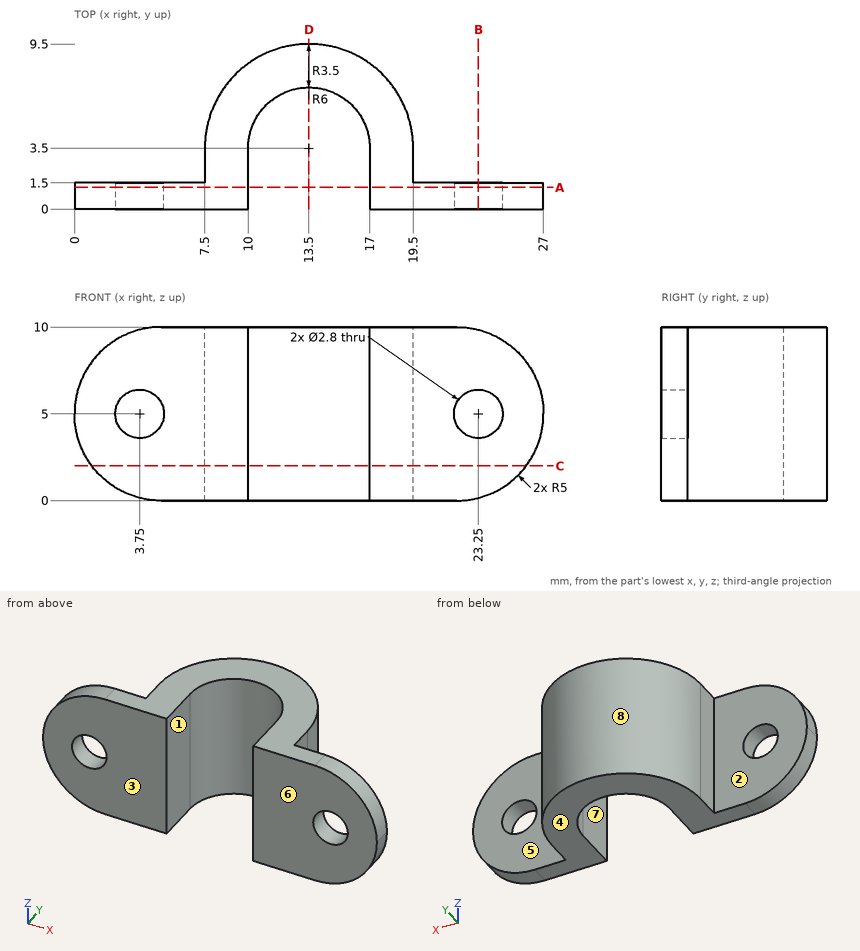
Part print with two shaded views. Sizes in mm from the minimum x, y, z corner. A direction names the side the tool comes from. Coordinates: 2 decimals unless noted, no trailing zeros. Order: outer loops, then holes, each group sorted by start corner. A loop starts at its lowest first (then second) coordinate and runs counter-clockwise, first axis right, second up. Notation, with made-up numbers: (2, 37.25) - (27, 37.25) arc R17 cw to (27, 66.25) - close; hole circle Ø3 at (-0.75, 87.5). An arc over 180 degrees is marked (long way). Write item = value, one per line. Start each with the question number.
1) Wall check: line 1 along X through (y, z) = (3, 4); line 2 along Y through (x, z) = (22, 2.25); line 3 along X through (y, z) = (5.25, 2.75). Give the ranges that are in metal, low to high. Write a range as from..to.
2) Two-plate mould, pull along X, no slides. Class the marked faces 6, 7 and 8: pulls with the +X half, pulls with the -X half, needs draft (parallel to the pull), parting line crosses it, or undercut.
3) Flat gauge pins, fed straight in: pin 1 Ø1 at (y, z) = (6.5, 8.5) entering from +X; pin 2 Ø1 at (x, z) = (9, 8) entering from +Y; pin 3 Ø1.6 at (y, z) = (3, 4.5) entering from -X. Where does each tip first touch, or does it go through?
4) Saw through at C-C on z = 2. Write the cut outline in (x, y), then the cut area to 3 significant figures.
5) Saw through at B-B on x = 23.25. Write the cut outline in (y, z).
6) Saw through at A-A on y = 1.25. Count the separate pieces of the cut face and the enclosed holes in it, then the cut area to 3 significant figures.
7) 3-axis set-ups, long thin cutter, end or side, ignore diameter. For the marked faces 1, 2, 3, 4 and 5: which of +Z, -Z, +X, -X, +Y, -Y reach the whole face in a straight line?
8) Saw through at D-D on x = 13.5. Write the cut outline in (y, z).
From the geometry:
q1.line_1 = 7.5..10, 17..19.5
q1.line_2 = 0..1.5
q1.line_3 = 7.76..10.47, 16.53..19.24
q2.face_6 = needs draft
q2.face_7 = undercut
q2.face_8 = parting line crosses it
q3.pin_1 = 18.95
q3.pin_2 = 7.97
q3.pin_3 = 7.5
q4.outline = (1, 0) - (10, 0) - (10, 3.5) arc R3.5 cw to (17, 3.5) - (17, 0) - (26, 0) - (26, 1.5) - (19.5, 1.5) - (19.5, 3.5) arc R6 ccw to (7.5, 3.5) - (7.5, 1.5) - (1, 1.5) - close
q4.area = 74.3 mm^2
q5.outline = (0, 0.16) - (1.5, 0.16) - (1.5, 3.6) - (0, 3.6) - close; (0, 6.4) - (1.5, 6.4) - (1.5, 9.84) - (0, 9.84) - close
q6.separate_pieces = 2
q6.enclosed_holes = 2
q6.area = 166 mm^2
q7.face_1 = +Z, -Z, -Y
q7.face_2 = +Z, -Z, -X, +Y
q7.face_3 = +Z, -Z, +X, -X, -Y
q7.face_4 = -Z, +X, -X, +Y, -Y
q7.face_5 = +Z, -Z, +X, +Y
q8.outline = (7, 0) - (9.5, 0) - (9.5, 10) - (7, 10) - close
